Work out the finished part from the listing and answer in its coordinate system (mm). A direction names the side the tool comes from. Give positions to 0.01 mm unless a question says otherwise; leave off trailing zeros. Order: outer loops, then holes, each group sorted by start corner. A loop starts at its lowest first (then second) coordinate and runs counter-clockwise, first axis right, second up. Notation, with made-up numbers: (51.25, 26.25) - (63.25, 26.25) arc R29 ccw to (63.25, 61.25) - close; hole circle Ø10 at (-14.75, 38.5). An arc over 180 degrees is marked (long way). Return JSON: item names as keys, results as strings. Group by question number.
from build123d import *

# Parameters (mm, degrees)
F0_W     = 25.4
F0_H     = 25.4
F1_DEPTH = 25.4
F2_W     = 6.35
F2_H     = 6.35
F2_R     = 3.175
F3_DEPTH = 2.54
F4_R     = 2.54


with BuildPart() as f1:
    # F0 (on Top) → F1 (new body)
    with BuildSketch(Plane.XY):
        Rectangle(F0_W, F0_H)
    extrude(amount=F1_DEPTH)

    # F2 (on face) → F3 (cut)
    with BuildSketch(Plane.XY.offset(25.4)):
        with Locations((-9.525, 9.525)):
            Rectangle(F2_W, F2_H)
        Circle(F2_R)
    extrude(amount=-F3_DEPTH, mode=Mode.SUBTRACT)

    # F4
    f4_edges = [f1.edges().sort_by_distance(p)[0] for p in [
        (-6.35, 6.35, 24.13),
    ]]
    fillet(f4_edges, radius=F4_R)


solid = f1.part
1. The part is cut by section A-A (x = 0). Give the vertices of the cut face in (y, z) (3 decimals), and give its area (3 significant figures).
2. A tool of negligible diameter and unlimited length cuts with its end or side. For faces 4 (the flat face through (-6.35, 11, 24)), 5 (the flat face through (0, -12.7, 13)), 6 (the flat face through (0, 0, 22.86)), from which of +Z, -Z, +X, -X, +Y, -Y can it reach the whole face along a straight path? Write none if from no direction.
3. Each of these flat-tipped pins is pushed along its axis until it touches: pin 1 (0.8 mm diameter, centred on x = -11.5, z = 24.5, fed in from +Y); pin 2 (5 mm diameter, centred on x = -10, y = 9, fed in from +Z). Where does it stop, or does it pass through?
4. Determine the mould class of faces 1 (the flat face through (-11, 6.35, 24)), 2 (the cylindrical face through (-7.114, 7.074, 24.112)), 3 (the cylindrical face through (-0.69, -3.1, 24.15)) for opening direction X: released by +X, released by -X, zero draft, split by the parting line, or undercut.
5. Consider probe 1 along Y at (x, z) = (0, 24.4) (3 decimals); probe 2 along Z at (x, y) = (-9.5, 10.25); probe 3 along Y at (x, z) = (0.5, 24.75). Determine where each line is inside the solid, lowest interval first. Write a range as from..to.
Answers:
{
 "1": {"outline": "(-12.7, 0) - (12.7, 0) - (12.7, 25.4) - (3.175, 25.4) - (3.175, 22.86) - (-3.175, 22.86) - (-3.175, 25.4) - (-12.7, 25.4) - close", "area": "629 mm^2"},
 "2": {"face 4": "+Z, -X, +Y", "face 5": "+Z, -Z, +X, -X, -Y", "face 6": "+Z"},
 "3": {"pin 1": "stops at y = 6.35", "pin 2": "stops at z = 22.86"},
 "4": {"face 1": "zero draft", "face 2": "released by -X", "face 3": "undercut"},
 "5": {"probe 1": "y = -12.7..-3.175, 3.175..12.7", "probe 2": "z = 0..22.86", "probe 3": "y = -12.7..-3.14, 3.14..12.7"}
}
